The listing builds one solid part. Answer for the finished solid, in the listing's coordinates (mm). A direction names the side the tool comes from. Coordinates: 2 decimals unless noted, no trailing zeros. Loops run counter-clockwise (first coordinate to the right, second up) from the corner with the lowest first, then second, coordinate; pieces in that order, holes last. Notation, with made-up numbers: M 65.25,2 L 112.25,2 A21 ccw 112.25,20 Z; hole C 51.5,27.25 d6. An arc over 180 degrees is marked long. Answer as a JSON object with one key per item and string values. Group by question number.
1. Straight lines are drawn through the part: L1, parallel to Z at x = 4, y = 4.5; L2, parallel to X at y = 6, z = -12.5; L3, parallel to Y at x = 11.25, z = -9.75. For each, find the intervals that lie inside material, in ascending order.
2. A cutting plane is placed at A-A on x = 5.5. Give the vertices of the cut face in (y, z), and give its area (3 significant figures).
3. Determine the mould class of faces 1 (the face through (13, 7, -26)), 2 (the face through (0, 5, -9)), 3 (the face through (-2, 3, -12)) for opening direction X: released by +X, released by -X, zero draft, split by the parting line, or undercut.
4. For faces 4 (the face through (24, 4, 0)), 5 (the face through (13, 1, 0)), 6 (the face through (13, 3, -26.5)), determine the directions among +Z, -Z, +X, -X, +Y, -Y from which every point of the face is accessible in a straight line to the end or side of a thin tool.
5. A cutting plane is placed at B-B on y = 0.5. Give the vertices of the cut face in (x, z).
6. Given pin 1 (3 mm diameter, centred on x = 7.5, z = -1.5, fed in from +Y); pin 2 (2 mm diameter, centred on x = 16.5, y = 2.5, fed in from +Z); pin 3 (1 mm diameter, centred on x = 19, z = -9, fed in from +Y), each flat-ended and moving along its own axis, determine where each tip first touches the part or whether it passes through.
7. A cutting plane is placed at C-C on y = 6.25. Give the vertices of the cut face in (x, z).
from build123d import *

# Parameters (mm, degrees)
BOSS_EXTRUDE1_DEPTH = 7
BOSS_EXTRUDE2_DEPTH = 2
SKETCH1_5_W         = 26
SKETCH1_5_H         = 18
BOSS_EXTRUDE3_DEPTH = 4


with BuildPart() as part:
    # Sketch1 → Boss-Extrude1 (new body)
    with BuildSketch(Plane(origin=(0, 0, 0), x_dir=(1, 0, 0), z_dir=(0, 1, 0))):
        Polygon((0, 0), (0, 6.5), (0, 24.5), (26, 24.5), (26, 6.5), (26, 0), (21.5, 0), (21.5, -2), (28, -2), (28, 26.5), (-2, 26.5), (-2, -2), (4.5, -2), (4.5, 0), align=None)
    extrude(amount=BOSS_EXTRUDE1_DEPTH)

    # Sketch1<3> → Boss-Extrude2 (add)
    with BuildSketch(Plane(origin=(0, 0, 0), x_dir=(1, 0, 0), z_dir=(0, 1, 0))):
        Polygon((26, 6.5), (0, 6.5), (0, 0), (4.5, 0), (21.5, 0), (26, 0), align=None)
    extrude(amount=BOSS_EXTRUDE2_DEPTH)

    # Sketch1<5> → Boss-Extrude3 (add)
    with BuildSketch(Plane(origin=(0, 0, 0), x_dir=(1, 0, 0), z_dir=(0, 1, 0))):
        with Locations((13, 15.5)):
            Rectangle(SKETCH1_5_W, SKETCH1_5_H)
    extrude(amount=BOSS_EXTRUDE3_DEPTH)


solid = part.part
From the geometry:
{
 "1": {"L1": "z = -26.5 to -24.5, 0 to 2", "L2": "x = -2 to 0, 26 to 28", "L3": "y = 0 to 4"},
 "2": {"outline": "M 0,-26.5 L 7,-26.5 L 7,-24.5 L 4,-24.5 L 4,-6.5 L 2,-6.5 L 2,0 L 0,0 Z", "area": "99.0 mm²"},
 "3": {"face 1": "zero draft", "face 2": "undercut", "face 3": "released by -X"},
 "4": {"face 4": "+Y", "face 5": "+Z, +Y, -Y", "face 6": "-Z, +X, -X, +Y, -Y"},
 "5": {"outline": "M -2,-26.5 L 28,-26.5 L 28,2 L 21.5,2 L 21.5,0 L 4.5,0 L 4.5,2 L -2,2 Z"},
 "6": {"pin 1": "stops at y = 2", "pin 2": "stops at z = 0", "pin 3": "stops at y = 4"},
 "7": {"outline": "M -2,-26.5 L 28,-26.5 L 28,2 L 21.5,2 L 21.5,0 L 26,0 L 26,-24.5 L 0,-24.5 L 0,0 L 4.5,0 L 4.5,2 L -2,2 Z"}
}
